```python
from build123d import *

# Parameters (mm, degrees)
F1_DEPTH  = 33
F3_DEPTH  = 5
F4_R      = 12.5
F5_DEPTH  = 4
F7_DEPTH  = 0.5
F8_R      = 11.5
F9_R      = 11.5
F11_DEPTH = 0.5
F13_DEPTH = 5
F12_R     = 1
F14_DEPTH = 1.5
F15_ANGLE = 180


with BuildPart() as f1:
    # F0 (on Front) → F1 (new body)
    with BuildSketch(Plane.XZ):
        Polygon((64.5, 38.5), (0, 38.5), (-64.5, 38.5), (-94.5, 38.5), (-94.5, 0), (-94.5, -38.5), (0, -38.5), (94.5, -38.5), (94.5, 0), (94.5, 38.5), align=None)
    extrude(amount=F1_DEPTH)

    # F2 (on face) → F3 (cut)
    with BuildSketch(Plane.XY.offset(38.5)):
        Polygon((-64.5, 0), (-94.5, 0), (-94.5, -16.5), (-94.5, -33), (-64.5, -33), (-64.5, -16.5), (-49.5, 0), align=None)
        Polygon((49.5, 0), (64.5, -16.5), (64.5, -33), (94.5, -33), (94.5, 0), (64.5, 0), align=None)
    extrude(amount=-F3_DEPTH, mode=Mode.SUBTRACT)

    # F4 (on face) → F5 (join)
    with BuildSketch(Plane.XY.offset(33.5)):
        with BuildLine():
            ThreePointArc((-66, -16.5), (-78.5, -4), (-91, -16.5))
            ThreePointArc((-91, -16.5), (-78.5, -29), (-66, -16.5))
        make_face()
        with Locations((78.5, -16.5)):
            Circle(F4_R)
    extrude(amount=F5_DEPTH)

    # F6 (on face) → F7 (cut)
    with BuildSketch(Plane.XY.offset(38.5)):
        Polygon((0, -1.5), (0, 0), (-49.5, 0), (-64.5, -16.5), (-64.5, -33), (0, -33), (0, -31), (-63, -31), (-63, -17.0799103121), (-48.8364451708, -1.5), align=None)
        Polygon((49.5, 0), (0, 0), (0, -1.5), (48.8364451708, -1.5), (63, -17.0799103121), (63, -31), (0, -31), (0, -33), (64.5, -33), (64.5, -16.5), align=None)
    extrude(amount=-F7_DEPTH, mode=Mode.SUBTRACT)

    # F8
    f8_edges = [f1.edges().sort_by_distance(p)[0] for p in [
        (-94.5, -33, -2.5),
    ]]
    fillet(f8_edges, radius=F8_R)

    # F9
    f9_edges = [f1.edges().sort_by_distance(p)[0] for p in [
        (-94.5, 0, -2.5),
        (94.5, 0, -2.5),
        (94.5, -33, -2.5),
    ]]
    fillet(f9_edges, radius=F9_R)

    # F10 (on Front) → F11 (cut)
    with BuildSketch(Plane.XZ):
        Polygon((69.7, -32.5), (69.7, 0), (69.7, 19.5), (0, 19.5), (-69.7, 19.5), (-69.7, 0), (-69.7, -32.5), (0, -32.5), align=None)
    extrude(amount=F11_DEPTH, mode=Mode.SUBTRACT)

    # F12 (on face) → F13 (cut)
    with BuildSketch(Plane(origin=(0, -0.5, 0), x_dir=(-1, 0, 0), z_dir=(0, 1, 0))):
        Polygon((-64.2, 15.5), (-64.2, 0), (-64.2, -28.5), (-48.5950261354, -28.5), (64.2, -28.5), (64.2, 15.5), (-38.0094833672, 15.5), align=None)
    extrude(amount=-F13_DEPTH, mode=Mode.SUBTRACT)

    # F12 (on face) → F14 (cut)
    with BuildSketch(Plane(origin=(0, -0.5, 0), x_dir=(-1, 0, 0), z_dir=(0, 1, 0))):
        with BuildLine():
            ThreePointArc((-66.2, 13), (-66.4928932188, 13.7071067812), (-67.2, 14))
            ThreePointArc((-67.2, 14), (-67.9071067812, 12.2928932188), (-66.2, 13))
        make_face()
        with BuildLine():
            ThreePointArc((-66.2, -6.5), (-66.4928932188, -5.7928932188), (-67.2, -5.5))
            ThreePointArc((-67.2, -5.5), (-67.9071067812, -7.2071067812), (-66.2, -6.5))
        make_face()
        with Locations((67.2, -26)):
            Circle(F12_R)
        with Locations((67.2, -6.5)):
            Circle(F12_R)
        with Locations((67.2, 13)):
            Circle(F12_R)
        with BuildLine():
            ThreePointArc((-66.2, -26), (-67.9071067812, -25.2928932188), (-67.2, -27))
            ThreePointArc((-67.2, -27), (-66.4928932188, -26.7071067812), (-66.2, -26))
        make_face()
    extrude(amount=-F14_DEPTH, mode=Mode.SUBTRACT)


with BuildPart() as f1_1:
    # F15: moved
    add(f1.part.rotate(Axis((83, 0, -2.5), (0, 0, 1)), F15_ANGLE))


with BuildPart() as f1_2:
    # F16: moved
    add(f1_1.part.moved(Location((-166, 0, 0))))


solid = f1_2.part
```
CAD build for the part. Positions are in the model's coordinates, mm. A direction names the side the tool comes from. Round coordinates to 2 decimals unless told otherwise and drop trailing zeros. Order: outer loops, then holes, each group sorted by start corner. A loop starts at its lowest first (then second) coordinate and runs counter-clockwise, first axis right, second up. Notation, with made-up numbers: (89.5, -15) - (114.5, -15) arc R14 ccw to (114.5, 0) - close; hole circle Ø5 at (88, 79). An arc over 180 degrees is marked (long way). Answer as CSV lines item,"result". Start each with the question number.
1. Saw through at D-D, the plane x = -47. Write the cut outline in (y, z).
2. Pin check, flat tips, straight feed: pin 1 (2 mm diameter, centred on y = 25, z = 6.5, fed in from -X) (3 decimals); pin 2 (0.6 mm diameter, centred on x = -8.5, y = 0.5, fed in from +Z); pin 3 (5 mm diameter, centred on y = 7, z = 10.5, fed in from +X). Stop position of each tip, or through.
3. Tool access for faces 5 (the face through (-78, 16, 37.5)), 6 (the face through (-1, 5.5, -6)), 7 (the face through (-56.895, 8.134, 35.782)), 8 (the face through (-64.5, 25, 36)), 9 (the face through (72, 5, 33.5)): list every direction of +Z, -Z, +X, -X, +Y, -Y with a clear straight run to the whole face (end or side of a thin tool).
4. Pull direction Z, two halves, no side cores. Call faces 1 (the face through (1, 16, -38.5)), 2 (the face through (-72, 5, 33.5)), 3 (the face through (91.22, 3.46, -3)), 4 (the face through (1, 3, 15.5)): +Z half, -Z half, draft (parallel to the pull), parting line (faces both ways), or undercut.
5. Saw through at A-A, the plane x = 78.5. Write the cut outline in (y, z).
6. Saw through at C-C, the plane y = 7.5. Write the cut outline in (x, z).
7. Saw through at B-B, the plane z = 9. Write the cut outline in (x, y), and give its area (3 significant figures).
8. Drill centre lines: L1, parallel to Z at x = -67.2, y = 1.5; L2, parallel to Z at x = -10, y = 5; L3, parallel to Y at x = -36.5, z = 5. Where is each one in solid material? Low to high. Write a range as [from, to].
Model answer:
1,outline,"(0, -38.5) - (33, -38.5) - (33, 38) - (31, 38) - (31, 38.5) - (1.5, 38.5) - (1.5, 38) - (0, 38) - (0, 19.5) - (0.5, 19.5) - (0.5, 15.5) - (5.5, 15.5) - (5.5, -28.5) - (0.5, -28.5) - (0.5, -32.5) - (0, -32.5) - close"
2,pin 1,"stops at x = -94.225"
2,pin 2,"stops at z = 38"
2,pin 3,"stops at x = 94.32"
3,face 5,"+Z, -X, +Y, -Y"
3,face 6,"-Y"
3,face 7,"+Z, -Y"
3,face 8,"+Z, +Y, -Y"
3,face 9,"+Z"
4,face 1,"-Z half"
4,face 2,"+Z half"
4,face 3,"draft"
4,face 4,"undercut"
5,outline,"(0, -38.5) - (33, -38.5) - (33, 33.5) - (29, 33.5) - (29, 37.5) - (4, 37.5) - (4, 33.5) - (0, 33.5) - close"
6,outline,"(-93.78, -38.5) - (93.78, -38.5) - (93.78, 33.5) - (87.17, 33.5) - (87.17, 37.5) - (69.83, 37.5) - (69.83, 33.5) - (56.32, 33.5) - (56.32, 38) - (54.29, 38) - (54.29, 38.5) - (-54.29, 38.5) - (-54.29, 38) - (-56.32, 38) - (-56.32, 33.5) - (-69.83, 33.5) - (-69.83, 37.5) - (-87.17, 37.5) - (-87.17, 33.5) - (-93.78, 33.5) - close"
7,outline,"(-94.5, 11.5) arc R11.5 ccw to (-83, 0) - (-69.7, 0) - (-69.7, 0.5) - (-64.2, 0.5) - (-64.2, 5.5) - (64.2, 5.5) - (64.2, 0.5) - (69.7, 0.5) - (69.7, 0) - (83, 0) arc R11.5 ccw to (94.5, 11.5) - (94.5, 21.5) arc R11.5 ccw to (83, 33) - (-83, 33) arc R11.5 ccw to (-94.5, 21.5) - close"
7,area,"5,410 mm²"
8,L1,"z = [-38.5, -27], [-25, -7.5], [-5.5, 12], [14, 33.5]"
8,L2,"z = [-38.5, -28.5], [15.5, 38.5]"
8,L3,"y = [5.5, 33]"
